Work out the finished part from the listing and answer in its coordinate system (mm). A direction names the side the tool comes from. Give positions to 0.01 mm unless a question says otherwise; leave off trailing zeros. Loops run counter-clockwise (first coordinate to the right, second up) from the corner with the lowest first, then second, coordinate; pieces in that order, holes last. Notation, with made-up numbers: M 35.5,37 L 50.5,37 A36 ccw 50.5,75 Z; hole C 14,18.5 d9. An arc over 180 degrees is marked long. Answer in a Markdown table with one row per item. Add a question column.
from build123d import *

# Parameters (mm, degrees)
SKETCH002_W         = 35.56
SKETCH002_H         = 2.54
PAD002_DEPTH        = 2.5
FILLET001_R         = 1
SKETCH003_W         = 1
SKETCH003_H         = 1
PAD003_DEPTH        = 7.5
LINEARPATTERN_COUNT = 14
LINEARPATTERN_PITCH = 2.54


with BuildPart() as part:
    # Sketch002 → Pad002 (new body)
    with BuildSketch(Plane.XY):
        with Locations((17.78, 0)):
            Rectangle(SKETCH002_W, SKETCH002_H)
    extrude(amount=-PAD002_DEPTH)

    # Fillet001
    fillet001_edges = [part.edges().sort_by_distance(p)[0] for p in [
        (35.56, 1.27, -1.25),
        (35.56, -1.27, -1.25),
        (0, 1.27, -1.25),
        (0, -1.27, -1.25),
    ]]
    fillet(fillet001_edges, radius=FILLET001_R)

    # Sketch003 (on Face5 of Fillet001) → Pad003 (join)
    with BuildSketch(Plane(origin=(0, 0, -2.5), x_dir=(1, 0, 0), z_dir=(0, 0, -1))):
        with Locations((1.27, 0)):
            Rectangle(SKETCH003_W, SKETCH003_H)
    pad003 = extrude(amount=PAD003_DEPTH)

    # LinearPattern: Pad003 ×14
    with Locations(*[(i * LINEARPATTERN_PITCH, 0, 0) for i in range(1, LINEARPATTERN_COUNT)]):
        add(pad003)


with BuildPart() as part_1:
    # Body001 placement: moved
    add(part.part.moved(Location((0, 7.62, 0))))


with BuildPart() as part_2:
    # Body002 placement: moved
    add(part_1.part.moved(Location((0, -15.24, 0))))


solid = part_2.part
(1) Section C-C, the plane y = -8.5 is taken. Determine the outline of the cut face in (x, z), and give its area (3 significant figures).
(2) Which of the six approach directions +Z, -Z, +X, -X, +Y, -Y give full straight-line access (tool end or side, diameter ignored) to faces 1 (the face through (6.85, -7.6, -6.2)), 2 (the face through (19, -7.12, -6)), 3 (the face through (27, -8.12, -6))?
(3) Each of these flat-tipped pins is pushed along its axis until it touches: P1, Ø0.5, axis at x = 16.5, z = -5.5, coming from the -Y side; P2, Ø1.5, axis at x = 16.5, z = -3.5, coming from the +Y side; P3, Ø4, axis at x = 8, z = -3, coming from the -Y side; P4, Ø0.5, axis at y = -7.5, z = -7, coming from the -X side. Where does it stop, or does it pass through?
(4) Section D-D, the plane y = -6.7 is taken. Determine the outline of the cut face in (x, z).
(5) Section B-B, the plane z = -6 is taken. State how many separate pieces and enclosed holes the cut face has, and give its area (3 significant figures).
(6) Consider line 1 along Z through (x, y) = (21, -8.5); line 2 along Y through (x, z) = (4, -7.5); line 3 along X through (y, z) = (-6.45, -1.5). Determine where each line is inside the solid, lowest interval first. Write a range as from..to.
(7) Section A-A, the plane x = 4 is taken. Determine the outline of the cut face in (y, z), and give its area (4 significant figures).
Numbers:
| question | item | result |
|---|---|---|
| 1 | outline | M 0.21,-2.5 L 35.35,-2.5 L 35.35,0 L 0.21,0 Z |
| 1 | area | 87.9 mm² |
| 2 | face 1 | -Z, +Y, -Y |
| 2 | face 2 | -Z, +X, -X, +Y |
| 2 | face 3 | -Z, +X, -X, -Y |
| 3 | P1 | stops at y = -8.12 |
| 3 | P2 | stops at y = -7.12 |
| 3 | P3 | stops at y = -8.89 |
| 3 | P4 | stops at x = 0.77 |
| 4 | outline | M 0.24,-2.5 L 35.32,-2.5 L 35.32,0 L 0.24,0 Z |
| 5 | separate pieces | 14 |
| 5 | enclosed holes | 0 |
| 5 | area | 14.0 mm² |
| 6 | line 1 | z = -2.5..0 |
| 6 | line 2 | y = -8.12..-7.12 |
| 6 | line 3 | x = 0.56..35 |
| 7 | outline | M -8.89,-2.5 L -8.12,-2.5 L -8.12,-10 L -7.12,-10 L -7.12,-2.5 L -6.35,-2.5 L -6.35,0 L -8.89,0 Z |
| 7 | area | 13.85 mm² |
